Model file for the job. Use its own axes, mm. Round coordinates to 2 decimals unless told otherwise and drop trailing zeros. Order: outer loops, then holes, each group sorted by start corner. A loop starts at its lowest first (then second) coordinate and runs counter-clockwise, first axis right, second up. Notation, with made-up numbers: (11, 65) - (28, 65) arc R30 cw to (28, 97) - close; hole circle Ø5 at (14.5, 83.25). An arc over 180 degrees is marked (long way). Put each result on its own line as item: value. Start each with the question number.
Item 1: Saw through at B-B on x = 56.25. List the corners of the cut face in (y, z), plus the area to 3 significant figures.
Item 2: Probe probe 1 along Z at (x, y) = (57, 0); probe 2 along Y at (x, z) = (56.5, 500); probe 3 along Z at (x, y) = (47.75, 4). List the from-to ranges inside material, lowest first.
Item 3: Saw through at C-C on x = 46. List the corners of the cut face in (y, z), plus the area to 3 significant figures.
Item 4: Pin check, flat tip, straight feed: pin 1 Ø8 at (x, z) = (47, 500.5) entering from +Y. Stop position of the tip, or through.
Item 5: Mould opens along Y. For faces 1 (the face through (50, -10, 505)), 2 (the face through (60, 0, 505)), 3 (the face through (56.041, 4.496, 500.198)) say: pulls with the +Y half, pulls with the -Y half, needs draft (parallel to the pull), parting line crosses it, or undercut.
Item 6: Saw through at D-D on y = 7.25. List the corners of the cut face in (x, z), plus the area to 3 significant figures.
Item 7: Saw through at A-A on z = 500. List the corners of the cut face in (x, y).
```python
from build123d import *

# Parameters (mm, degrees)
SKETCH_W            = 20
SKETCH_H            = 20
PAD_DEPTH           = 10
HOLE_D              = 5
HOLE_DEPTH          = 25
HOLE_CBORE_D        = 9
HOLE_CBORE_DEPTH    = 20
HOLE001_D           = 5
HOLE001_DEPTH       = 25
HOLE001_CBORE_D     = 9
HOLE001_CBORE_DEPTH = 20


with BuildPart() as part:
    # Sketch → Pad (new body, symmetric)
    with BuildSketch(Plane.XY):
        Rectangle(SKETCH_W, SKETCH_H)
    extrude(amount=PAD_DEPTH, both=True)

    # Hole
    with Locations(Plane.XZ.offset(10)):
        with Locations((0, 0)):
            CounterBoreHole(HOLE_D / 2, HOLE_CBORE_D / 2, HOLE_CBORE_DEPTH, depth=HOLE_DEPTH)

    # Hole001
    with Locations(Plane(origin=(-10, 0, 0), x_dir=(0, -1, 0), z_dir=(-1, 0, 0))):
        with Locations((0, 0)):
            CounterBoreHole(HOLE001_D / 2, HOLE001_CBORE_D / 2, HOLE001_CBORE_DEPTH, depth=HOLE001_DEPTH)


with BuildPart() as part_1:
    # Body placement: moved
    add(part.part.moved(Location((50, 0, 500))))


solid = part_1.part
```
Results found:
1. outline: (-10, 490) - (10, 490) - (10, 510) - (-10, 510) - close; hole circle Ø9 at (0, 500)
1. area: 336 mm²
2. probe 1: z = 490 to 495.5, 504.5 to 510
2. probe 2: y = -10 to -4.5, 4.5 to 10
2. probe 3: z = 490 to 496.1, 503.9 to 510
3. outline: (-10, 490) - (10, 490) - (10, 497.94) - (4, 497.94) arc R4.5 cw to (-4, 497.94) - (-10, 497.94) - close; (-10, 502.06) - (-4, 502.06) arc R4.5 cw to (4, 502.06) - (10, 502.06) - (10, 510) - (-10, 510) - close
3. area: 290 mm²
4. pin 1: stops at y = 10
5. face 1: pulls with the -Y half
5. face 2: needs draft
5. face 3: undercut
6. outline: (40, 490) - (60, 490) - (60, 510) - (40, 510) - close; hole circle Ø9 at (50, 500)
6. area: 336 mm²
7. outline: (40, -10) - (45.5, -10) - (45.5, -4.5) - (40, -4.5) - close; (40, 4.5) - (45.5, 4.5) - (45.5, 10) - (40, 10) - close; (54.5, -10) - (60, -10) - (60, -4.5) - (54.5, -4.5) - close; (54.5, 4.5) - (60, 4.5) - (60, 10) - (54.5, 10) - close
